Autodesk Fusion 360 part; units mm, degrees
sketch "스케치1" plane through (0, 0, 0) normal (0, 0, 1) x (1, 0, 0)
  line L0 (10, 24) -> (-10, 24)
  line L1 (-10, 24) -> (-10, -24)
  line L2 (-10, -24) -> (10, -24)
  line L3 (10, -24) -> (10, 24)
  line L4 (10, 24) -> (-10, -24) construction
  line L5 (-10, 24) -> (10, -24) construction
  circle A0 centre (0, 0) radius 2.65
  line L6 (0, 0) -> (0, 12)
  circle A1 centre (0, 12) radius 1.6
  line L7 (0, 0) -> (0, -12)
  circle A2 centre (0, -12) radius 1.6
  line L8 (10, 24) -> (11, 24)
  line L9 (11, 24) -> (11, -24)
  line L10 (11, -24) -> (10, -24)
  line L11 (10, -24) -> (10, 24)
  line L12 (11, 24) -> (14, 24)
  line L13 (14, 24) -> (14, -24)
  line L14 (14, -24) -> (11, -24)
  line L15 (11, -24) -> (11, 24)
  line L16 (10, -6) -> (14, -6)
  dimension "d1" = 20
  dimension "d2" = 48
  dimension "d3" = 5.3
  dimension "d4" = 12
  dimension "d5" = 3.2
  dimension "d6" = 12
  dimension "d7" = 3.2
  dimension "d12" = 3
extrude "돌출1" add sketch "스케치1" along normal blind 5 contours L0 L1 L2 L3 L11 | L3 L8 L9 L11 L15 L16 | L3 L9 L10 L11 L15 L16
extrude "돌출2" add sketch "스케치1" along normal blind 2.8 contours A2 | A1
extrude "돌출3" add sketch "스케치1" along normal blind 15 contours L9 L12 L13 L15 L16 | L9 L13 L14 L15 L16
Input: part model. Units: mm. Frame: model coordinates. A direction names the side the tool comes from. Coordinates: 2 decimals unless noted, no trailing zeros. Loops run counter-clockwise (first coordinate to the right, second up) from the corner with the lowest first, then second, coordinate; pieces in that order, holes last. Notation, with made-up numbers: (2.25, -35.5) - (29.25, -35.5) arc R25 cw to (29.25, -16.5) - close; hole circle Ø4 at (60.5, -23.75). An arc over 180 degrees is marked (long way). Answer in a Markdown table with one row per item.
(1) Mould query, pull axis Y, two halves, no side actions, for faces 1 (the face through (5, 24, 4)), 2 (the face through (2.45, 1.01, 2.46)), 3 (the face through (11, 0, 10)), 4 (the face through (-0.208, -13.586, 3.885)). Classes: pulls with the +Y half, pulls with the -Y half, needs draft (parallel to the pull), parting line crosses it, or undercut.
Model answer:
| item | result |
|---|---|
| face 1 | pulls with the +Y half |
| face 2 | undercut |
| face 3 | needs draft |
| face 4 | undercut |
(2) Material intervals for L1, parallel to Y at x = 0, z = 3.35; L2, parallel to Y at x = 0, z = 1.2; L3, parallel to X at y = 12, z = 3.8, sorted ascending. Write a range as from..to.
Model answer:
| item | result |
|---|---|
| L1 | y = -24..-13.6, -10.4..-2.65, 2.65..10.4, 13.6..24 |
| L2 | y = -24..-2.65, 2.65..24 |
| L3 | x = -10..-1.6, 1.6..14 |
(3) Cut plane B-B on x = 0. Output: boundary loops of the cut face in (y, z), plus the area to 3 significant figures.
Model answer:
| item | result |
|---|---|
| outline | (-24, 0) - (-2.65, 0) - (-2.65, 5) - (-10.4, 5) - (-10.4, 2.8) - (-13.6, 2.8) - (-13.6, 5) - (-24, 5) - close; (2.65, 0) - (24, 0) - (24, 5) - (13.6, 5) - (13.6, 2.8) - (10.4, 2.8) - (10.4, 5) - (2.65, 5) - close |
| area | 199 mm² |
(4) Pin query (flat end, axial travel): P1, Ø6.5, axis at x = -2.5, y = -4.5, coming from the +Z side; P2, Ø2, axis at y = -4.5, z = 12.5, coming from the -X side; P3, Ø1.6, axis at x = -0.5, y = 12, coming from the +Z side. Return the tip coordinate at first contact, or that it passes through.
Model answer:
| item | result |
|---|---|
| P1 | stops at z = 5 |
| P2 | stops at x = 11 |
| P3 | stops at z = 2.8 |
(5) Cut plane A-A on y = 0. Output: boundary loops of the cut face in (x, z), plus the area to 4 significant figures.
Model answer:
| item | result |
|---|---|
| outline | (-10, 0) - (-2.65, 0) - (-2.65, 5) - (-10, 5) - close; (2.65, 0) - (14, 0) - (14, 15) - (11, 15) - (11, 5) - (2.65, 5) - close |
| area | 123.5 mm² |
(6) Set-up query: faces 5 (the face through (14, 0, 7)), 6 (the face through (-0.35, 13.56, 3.88)), 7 (the face through (3, 0, 5)). Return all of +Z, -Z, +X, -X, +Y, -Y with unobstructed straight access to the full face (end or side cutting, diameter ignored); none if empty.
Model answer:
| item | result |
|---|---|
| face 5 | +Z, -Z, +X, +Y, -Y |
| face 6 | +Z |
| face 7 | +Z, -X, +Y, -Y |
(7) Cut plane C-C on y = -12. Output: boundary loops of the cut face in (x, z).
Model answer:
| item | result |
|---|---|
| outline | (-10, 0) - (14, 0) - (14, 15) - (11, 15) - (11, 5) - (1.6, 5) - (1.6, 2.8) - (-1.6, 2.8) - (-1.6, 5) - (-10, 5) - close |
(8) Cut plane D-D on x = 9.75. Output: boundary loops of the cut face in (y, z).
Model answer:
| item | result |
|---|---|
| outline | (-24, 0) - (24, 0) - (24, 5) - (-24, 5) - close |
